Can you work these out from the model? Positions are in its coordinate system, mm. Face numbers are marked on the shaded views. A direction names the side the tool comes from. Give positions to 0.01 mm unless a question says otherwise; leave off trailing zeros. Order: outer loops, then holes, each group sorted by start corner. A loop starts at its lowest first (then second) coordinate and runs counter-clockwise, first axis right, second up. Notation, with made-up numbers: (26.25, 11.25) - (74.25, 11.25) arc R23 cw to (74.25, 38.25) - close; hole circle Ø10 at (58.25, 46.5). An arc over 180 degrees is marked (long way). Write each question's results on one line, items separated by ' | '. Start each with the question number.
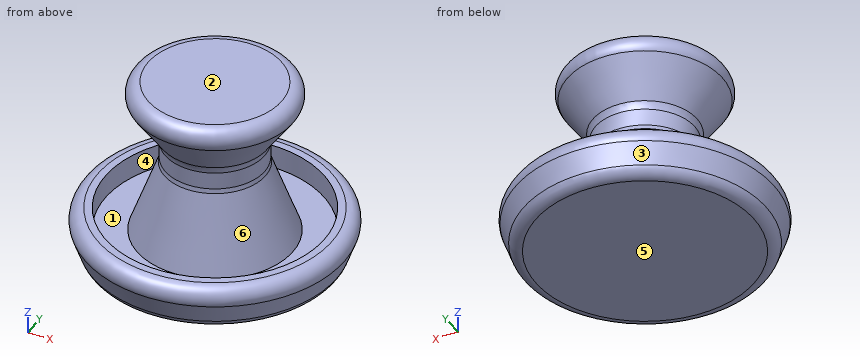
from build123d import *

# Parameters (mm, degrees)
F2_R = 5
F3_R = 5
F4_R = 5


with BuildPart() as f1:
    # F0 (on Front) → F1 (revolve)
    with BuildSketch(Plane.XZ):
        Polygon((-13.5948596994, -38), (31.4051403006, -38), (31.4051403006, 32), (-3.5948596994, 32), (12.5099136795, 9), (12.5099136795, 0), (1.8536760838, -29), (-10.1463239162, -29), (-10.1463239162, -20), (-20.1463239162, -20), align=None)
    revolve(axis=Axis((31.4051403006, 0, -3), (0, 0, -1)))

    # F2
    f2_edges = [f1.edges().sort_by_distance(p)[0] for p in [
        (66.40514, 0, 32),
        (82.956605, 0, -20),
    ]]
    fillet(f2_edges, radius=F2_R)

    # F3
    f3_edges = [f1.edges().sort_by_distance(p)[0] for p in [
        (50.300367, 0, 0),
        (50.300367, 0, 9),
    ]]
    fillet(f3_edges, radius=F3_R)

    # F4
    f4_edges = [f1.edges().sort_by_distance(p)[0] for p in [
        (76.40514, 0, -38),
    ]]
    fillet(f4_edges, radius=F4_R)


solid = f1.part
Q1. If I drill on probe 1 along Y at (x, z) = (50.5, -28); probe 2 along Z at (x, y) = (13, -27); probe 3 along Z at (x, y) = (10.5, -15.5), over which ranges is the centre line in solid material (lowest first)? Write a range as from..to.
Q2. Which directions (+Z, -Z, +X, -X, +Y, -Y) give clear straight access to the entire face, cutting with the end or side of a thin tool? Please do the marked faces 4, 5 and 6.
Q3. If we section it at B-B (z = -7): Please give me the cut outline in (x, y).
Q4. If we section it at A-A (z = 20): Please give me the cut outline in (x, y), plus the area to 3 significant figures.
Q5. Will these pins go through, and if not, where does the flat tip stop? P1, Ø12, axis at x = 34, z = -5.5, coming from the +Y side; P2, Ø6, axis at y = -7.5, z = 11, coming from the -X side; P3, Ø12, axis at y = -8, z = -12, coming from the -X side.
Q6. Thinking about a two-plate mould opening in X: for the marked faces 1, 2 and 3, which applies, released by +X, released by -X, zero draft, split by the parting line, or undercut?
Findings below:
1) probe 1: y = -44.73..-36.9, -22.07..22.07, 36.9..44.73 | probe 2: z = -38..-29 | probe 3: z = -38..-19.4, 19.18..31.96
2) face 4: +Z | face 5: -Z, +X, -X, +Y, -Y | face 6: none
3) outline: circle Ø42.93 at (31.41, 0)
4) outline: circle Ø53.2 at (31.41, 0) | area: 2,220 mm2
5) P1: stops at y = 23.04 | P2: stops at x = 10.1 | P3: stops at x = 6.69
6) face 1: undercut | face 2: zero draft | face 3: split by the parting line
